from build123d import *

# Parameters (mm, degrees)
SKETCH1_R           = 1.5
BOSS_EXTRUDE2_DEPTH = 2.54
BOSS_EXTRUDE3_DEPTH = 19.05
BOSS_EXTRUDE6_DEPTH = 19.05
SKETCH4_R           = 1
CUT_EXTRUDE1_DEPTH  = 158.597711186
FILLET1_R           = 6.35


with BuildPart() as part:
    # Sketch1 → Boss-Extrude2 (new body)
    with BuildSketch(Plane(origin=(0, 0, 0), x_dir=(1, 0, 0), z_dir=(0, 1, 0))):
        Polygon((-93.521103592, -81.172331094), (-106.459273851, -63.257941504), (-124.37366344, -76.196111763), (-111.435493182, -94.110501353), align=None)
        with Locations(Location((-114.3, -82.55, 0), (0, 0, 270))):
            Circle(SKETCH1_R, mode=Mode.SUBTRACT)
    extrude(amount=BOSS_EXTRUDE2_DEPTH)

    # Sketch2 → Boss-Extrude3 (add)
    with BuildSketch(Plane(origin=(0, 2.54, 0), x_dir=(1, 0, 0), z_dir=(0, 1, 0))):
        Polygon((-106.459273851, -63.257941504), (-124.37366344, -76.196111763), (-111.435493182, -94.110501353), (-93.521103592, -81.172331094), align=None)
        with BuildLine():
            Line((-106.888258276, -65.91764494), (-121.713960005, -76.625096188))
            Line((-121.713960005, -76.625096188), (-118.022197338, -81.736767574))
            ThreePointArc((-118.022197338, -81.736767574), (-117.38868786, -84.78071901), (-114.698271424, -86.339126532))
            Line((-114.698271424, -86.339126532), (-111.006508757, -91.450797917))
            Line((-111.006508757, -91.450797917), (-96.180807028, -80.743346669))
            Line((-96.180807028, -80.743346669), (-106.888258276, -65.91764494))
        make_face(mode=Mode.SUBTRACT)
    extrude(amount=BOSS_EXTRUDE3_DEPTH)

    # Sketch3 → Boss-Extrude6 (add)
    with BuildSketch(Plane(origin=(0, 21.59, 0), x_dir=(1, 0, 0), z_dir=(0, 1, 0))):
        Polygon((-121.713960005, -76.625096188), (-121.188174492, -77.353106899), (-109.675394227, -79.210006941), (-111.53229427, -90.722787207), (-111.006508757, -91.450797917), (-110.278498046, -90.925012404), (-108.421598003, -79.412232139), (-96.908817738, -81.269132182), (-96.180807028, -80.743346669), (-96.706592541, -80.015335958), (-108.219372806, -78.158435915), (-106.362472763, -66.64565565), (-106.888258276, -65.91764494), (-107.616268987, -66.443430453), (-109.473169029, -77.956210718), (-120.985949295, -76.099310675), align=None)
    extrude(amount=-BOSS_EXTRUDE6_DEPTH)

    # Sketch4 → Cut-Extrude1 (cut, through all)
    with BuildSketch(Plane(origin=(6.469085129, 0, 8.957194795), x_dir=(0.8106792283998809, 0, -0.5854905538443587), z_dir=(0.5854905538443586, 0, 0.8106792283998808))):
        with Locations(Location((-134.390249188, 12.7, 0), (0, 0, 90))):
            Circle(SKETCH4_R)
    extrude(amount=-CUT_EXTRUDE1_DEPTH, mode=Mode.SUBTRACT)

    # Fillet1
    fillet1_edges = [part.edges().sort_by_distance(p)[0] for p in [
        (-103.593657892, 2.54, 86.097072293),
        (-114.301109141, 2.54, 71.271370564),
    ]]
    fillet(fillet1_edges, radius=FILLET1_R)


solid = part.part
Part model, mm, in its own coordinate system. A direction names the side the tool comes from. Give positions to 0.01 mm unless a question says otherwise; leave off trailing zeros. Loops run counter-clockwise (first coordinate to the right, second up) from the corner with the lowest first, then second, coordinate; pieces in that order, holes last.
(1) 3-axis set-ups, long thin cutter, end or side, ignore diameter. For faces 4 (the cylindrical face through (-104.149, 5.305, 85.131)), 5 (the cylindrical face through (-102.31, 13.16, 86.36)): which of +Z, -Z, +X, -X, +Y, -Y reach the whole face in a straight line?
Return value:
face 4: +Y
face 5: none
(2) Pin check, flat tips, straight feed: pin 1 (4 mm diameter, centred on y = 15.5, z = 85, fed in from -X); pin 2 (2 mm diameter, centred on y = 17.5, z = 87.5, fed in from +X); pin 3 (1.5 mm diameter, centred on x = -103.5, y = 15.5, fed in from -Z). Stop position of each tip, or through.
Return value:
pin 1: stops at x = -119.46
pin 2: stops at x = -100.9
pin 3: stops at z = 66.32
(3) Pull direction Z, two halves, no side cores. Call faces 1 (the flat face through (-117.995, 10.644, 85.028)), 2 (the flat face through (-99.9, 10.64, 72.34)), 3 (the flat face through (-115.51, 12.2, 78.27)): pulls with the +Z half, pulls with the -Z half, needs draft (parallel to the pull), parting line crosses it, or undercut.
Return value:
face 1: pulls with the +Z half
face 2: pulls with the -Z half
face 3: undercut
(4) Band-saw the part on B-B (y = 6.75). Write the cut outline in (x, z).
Return value:
outline: (-124.37, 76.2) - (-106.46, 63.26) - (-93.52, 81.17) - (-111.44, 94.11) - close; hole (-121.19, 77.35) - (-109.68, 79.21) - (-111.53, 90.72) - (-114.7, 86.34) arc R3.81 ccw to (-118.02, 81.74) - close; hole (-120.47, 76.18) - (-107.7, 66.96) - (-109.47, 77.96) - close; hole (-110.19, 90.41) - (-108.42, 79.41) - (-97.43, 81.19) - close; hole (-108.22, 78.16) - (-106.36, 66.65) - (-96.71, 80.02) - close
(5) Drill centre lines: line 1 along X through (y, z) = (20, 75); line 2 along X through (y, z) = (13.25, 69); line 3 along Z through (x, y) = (-115.5, 3.25). Where is each one in solid material? Low to high.
Return value:
line 1: x = -122.72 to -119.46, -109 to -107.71, -100.33 to -97.98
line 2: x = -114.41 to -111.16, -108.03 to -106.74, -104.66 to -102.31
line 3: z = 69.79 to 76.37, 76.98 to 78.27, 86.17 to 88.48
(6) Band-saw the part on C-C (z = 65). Write the cut outline in (x, y).
Return value:
outline: (-108.87, 0) - (-105.2, 0) - (-105.2, 21.59) - (-108.87, 21.59) - close
(7) Band-saw the part on A-A (y = 19). Write the cut outline in (x, z), and give its area (3 significant figures).
Return value:
outline: (-124.37, 76.2) - (-106.46, 63.26) - (-93.52, 81.17) - (-111.44, 94.11) - close; hole (-121.19, 77.35) - (-109.68, 79.21) - (-111.53, 90.72) - (-114.7, 86.34) arc R3.81 ccw to (-118.02, 81.74) - close; hole (-120.99, 76.1) - (-107.62, 66.44) - (-109.47, 77.96) - close; hole (-110.28, 90.93) - (-108.42, 79.41) - (-96.91, 81.27) - close; hole (-108.22, 78.16) - (-106.36, 66.65) - (-96.71, 80.02) - close
area: 211 mm2
